CAD build for the part. Positions are in the model's coordinates, mm. Face numbers are marked on the shaded views. A direction names the side the tool comes from. Give positions to 0.01 mm unless a question says otherwise; leave off trailing zeros. Order: outer loops, then holes, each group sorted by start corner. A loop starts at its lowest first (then second) coordinate and runs counter-clockwise, first axis right, second up.
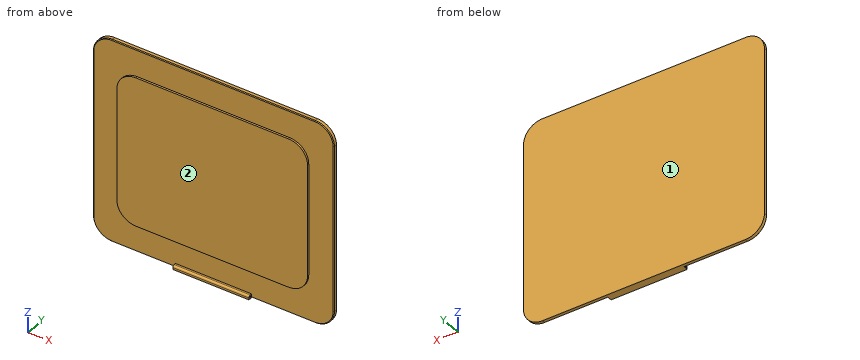
```python
from build123d import *

# Parameters (mm, degrees)
BOSS_EXTRUDE1_DEPTH            = 5
CHAMFER1_SIZE                  = 2
SKETCH4_W                      = 200
SKETCH4_H                      = 10
BOSS_EXTRUDE3_DEPTH            = 20
CUT_EXTRUDE1_REACH             = 318
SKETCH5_R                      = 2
CUT_EXTRUDE1_DIRECTION_2_REACH = 318
BOSS_EXTRUDE4_DEPTH            = 5


with BuildPart() as part:
    # Sketch1 → Boss-Extrude1 (new body, symmetric)
    with BuildSketch(Plane(origin=(0, 0, 0), x_dir=(1, 0, 0), z_dir=(0, 1, 0))):
        with BuildLine():
            Line((-266, 272.5), (266, 272.5))
            ThreePointArc((266, 272.5), (301.355339059, 257.855339059), (316, 222.5))
            Line((316, 222.5), (316, -222.5))
            ThreePointArc((316, -222.5), (301.355339059, -257.855339059), (266, -272.5))
            Line((266, -272.5), (-266, -272.5))
            ThreePointArc((-266, -272.5), (-301.355339059, -257.855339059), (-316, -222.5))
            Line((-316, -222.5), (-316, 222.5))
            ThreePointArc((-316, 222.5), (-301.355339059, 257.855339059), (-266, 272.5))
        make_face()
    extrude(amount=BOSS_EXTRUDE1_DEPTH, both=True)

    # Chamfer1
    chamfer1_edges = [part.edges().sort_by_distance(p)[0] for p in [
        (316, -5, 0),
        (301.355339059, -5, 257.855339059),
        (0, -5, 272.5),
        (-301.355339059, -5, 257.855339059),
        (-316, -5, 0),
        (-301.355339059, -5, -257.855339059),
        (0, -5, -272.5),
        (301.355339059, -5, -257.855339059),
    ]]
    chamfer(chamfer1_edges, length=CHAMFER1_SIZE)

    # Sketch4 → Boss-Extrude3 (add)
    with BuildSketch(Plane(origin=(0, 5, 0), x_dir=(1, 0, 0), z_dir=(0, 1, 0))):
        with Locations((0, 267.5)):
            Rectangle(SKETCH4_W, SKETCH4_H)
    extrude(amount=-BOSS_EXTRUDE3_DEPTH)

    # Sketch5 → Cut-Extrude1 (cut, up to next)
    with BuildSketch(Plane(origin=(0, 0, 0), x_dir=(0, 0, -1), z_dir=(1, 0, 0)), mode=Mode.PRIVATE) as cut_extrude1_sk1:
        with Locations((267.5, -9.996889361)):
            Circle(SKETCH5_R)
    cut_extrude1_tool1 = extrude(cut_extrude1_sk1.sketch, amount=-CUT_EXTRUDE1_REACH, mode=Mode.PRIVATE) & part.part
    add(cut_extrude1_tool1.solids().sort_by_distance((0, -9.996889, -267.5))[0], mode=Mode.SUBTRACT)
    # Sketch5 → Cut-Extrude1 (cut, up to next)
    with BuildSketch(Plane(origin=(0, 0, 0), x_dir=(0, 0, -1), z_dir=(1, 0, 0)), mode=Mode.PRIVATE) as cut_extrude1_sk2:
        with BuildLine():
            Line((267.5, -15), (267.5, -14.996889361))
            ThreePointArc((267.5, -14.996889361), (263.964466094, -13.532423267), (262.5, -9.996889361))
            Line((262.5, -9.996889361), (262.5, -15))
            Line((262.5, -15), (267.5, -15))
        make_face()
    cut_extrude1_tool2 = extrude(cut_extrude1_sk2.sketch, amount=-CUT_EXTRUDE1_REACH, mode=Mode.PRIVATE) & part.part
    add(cut_extrude1_tool2.solids().sort_by_distance((0, -13.883283, -263.620838))[0], mode=Mode.SUBTRACT)

    # Sketch5 → Cut-Extrude1 direction 2 (cut, up to next)
    with BuildSketch(Plane(origin=(0, 0, 0), x_dir=(0, 0, -1), z_dir=(1, 0, 0)), mode=Mode.PRIVATE) as cut_extrude1_direction_2_sk1:
        with Locations((267.5, -9.996889361)):
            Circle(SKETCH5_R)
    cut_extrude1_direction_2_tool1 = extrude(cut_extrude1_direction_2_sk1.sketch, amount=CUT_EXTRUDE1_DIRECTION_2_REACH, mode=Mode.PRIVATE) & part.part
    add(cut_extrude1_direction_2_tool1.solids().sort_by_distance((0, -9.996889, -267.5))[0], mode=Mode.SUBTRACT)
    # Sketch5 → Cut-Extrude1 direction 2 (cut, up to next)
    with BuildSketch(Plane(origin=(0, 0, 0), x_dir=(0, 0, -1), z_dir=(1, 0, 0)), mode=Mode.PRIVATE) as cut_extrude1_direction_2_sk2:
        with BuildLine():
            Line((267.5, -15), (267.5, -14.996889361))
            ThreePointArc((267.5, -14.996889361), (263.964466094, -13.532423267), (262.5, -9.996889361))
            Line((262.5, -9.996889361), (262.5, -15))
            Line((262.5, -15), (267.5, -15))
        make_face()
    cut_extrude1_direction_2_tool2 = extrude(cut_extrude1_direction_2_sk2.sketch, amount=CUT_EXTRUDE1_DIRECTION_2_REACH, mode=Mode.PRIVATE) & part.part
    add(cut_extrude1_direction_2_tool2.solids().sort_by_distance((0, -13.883283, -263.620838))[0], mode=Mode.SUBTRACT)

    # Sketch6 → Boss-Extrude4 (add)
    with BuildSketch(Plane.XZ.offset(5)):
        with BuildLine():
            Line((-200, 200), (200, 200))
            ThreePointArc((200, 200), (235.355339059, 185.355339059), (250, 150))
            Line((250, 150), (250, -150))
            ThreePointArc((250, -150), (235.355339059, -185.355339059), (200, -200))
            Line((200, -200), (-200, -200))
            ThreePointArc((-200, -200), (-235.355339059, -185.355339059), (-250, -150))
            Line((-250, -150), (-250, 150))
            ThreePointArc((-250, 150), (-235.355339059, 185.355339059), (-200, 200))
        make_face()
    extrude(amount=BOSS_EXTRUDE4_DEPTH)


solid = part.part
```
Item 1: Tool access for the marked faces 1 and 2: list every direction of +Z, -Z, +X, -X, +Y, -Y with a clear straight run to the whole face (end or side of a thin tool).
Item 2: Slice it at C-C (x = 243). Give the cut face in (y, z), and give its area (3 significant figures).
Item 3: Slice it at A-A (z = 140). Give the cut face in (x, y), and give its area (3 significant figures).
Item 4: Drop flat-ended pins along their axis: pin 1 Ø5.5 at (y, z) = (-7, 70) entering from +X; pin 2 Ø10 at (x, z) = (-150.5, 41) entering from -Y; pin 3 Ø4 at (x, y) = (-116, -8) entering from +Z; pin 4 Ø8 at (y, z) = (-4.5, 172) entering from +X. Give the stop position or say it passes through.
Item 5: Wall check: L1, parallel to Y at x = 14.5, z = -267.5; L2, parallel to Z at x = -56.5, y = -8.25; L3, parallel to Y at x = 27, z = -267. Give the ranges that are in metal, low to high.
A:
1. face 1: +Z, -Z, +X, -X, +Y
1. face 2: +Z, +X, -X, -Y
2. outline: (-10, -175.51) - (-5, -175.51) - (-5, -270.5) - (-3, -272.5) - (5, -272.5) - (5, 272.5) - (-3, 272.5) - (-5, 270.5) - (-5, 175.51) - (-10, 175.51) - close
2. area: 7,200 mm2
3. outline: (-316, -3) - (-314, -5) - (-250, -5) - (-250, -10) - (250, -10) - (250, -5) - (314, -5) - (316, -3) - (316, 5) - (-316, 5) - close
3. area: 8,820 mm2
4. pin 1: stops at x = 314.75
4. pin 2: stops at y = -10
4. pin 3: stops at z = 200
4. pin 4: stops at x = 316
5. L1: y = -15 to -12, -8 to 5
5. L2: z = -272.5 to -268.47, -266.53 to -262.5, -200 to 200
5. L3: y = -14.97 to -11.93, -8.06 to 5
